Part model, mm, in its own coordinate system. Coordinates: 2 decimals unless noted, no trailing zeros. Loops run counter-clockwise (first coordinate to the right, second up) from the corner with the lowest first, then second, coordinate; pieces in that order, holes last. Notation, with made-up numbers: (19, 84) -> (78, 84) arc R26 ccw to (78, 108) -> close; hole circle Ø1 at (-21.5, 89.25). An arc over 180 degrees is marked (long way). One line per question, with ' | ' between items. Start each with the question number.
1) Cut at B-B (z = 2.25). List the corners of the cut face in (x, y).
2) Probe L1, parallel to Y at x = 27.5, z = 6; L2, parallel to Z at x = 4, y = -88; L3, parallel to Y at x = -20.5, z = 8.25. List the from-to ranges inside material, lowest first. Write a range as from..to.
3) Drop flat-ended pins along their axis: pin 1 (1 mm diameter, centred on x = 6, z = 2, fed in from -Y); pin 2 (4 mm diameter, centred on x = -13, y = -91, fed in from +Z). Give the stop position or say it passes through.
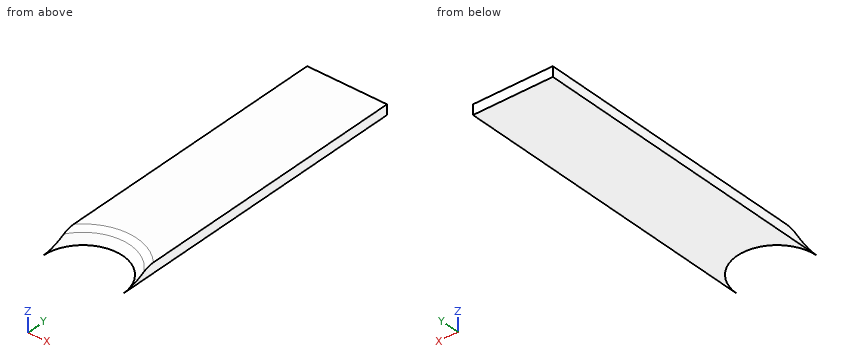
from build123d import *

# Parameters (mm, degrees)
SKETCH1_W           = 80
SKETCH1_H           = 360
BOSS_EXTRUDE1_DEPTH = 10
CUT_EXTRUDE1_DEPTH  = 10
CHAMFER2_SIZE       = 10
FILLET1_R           = 10


with BuildPart() as part:
    # Sketch1 → Boss-Extrude1 (new body)
    with BuildSketch(Plane.XY):
        Rectangle(SKETCH1_W, SKETCH1_H)
    extrude(amount=BOSS_EXTRUDE1_DEPTH)

    # Sketch2 → Cut-Extrude1 (cut)
    with BuildSketch(Plane.XY.offset(10)):
        with BuildLine():
            Line((-40, -135), (-40, -180))
            Line((-40, -180), (40, -180))
            Line((40, -180), (40, -135))
            ThreePointArc((40, -135), (0, -95), (-40, -135))
        make_face()
    extrude(amount=-CUT_EXTRUDE1_DEPTH, mode=Mode.SUBTRACT)

    # Chamfer2
    chamfer2_edges = [part.edges().sort_by_distance(p)[0] for p in [
        (0, -95, 10),
    ]]
    chamfer(chamfer2_edges, length=CHAMFER2_SIZE - 0.0001)  # a hair under: the kernel refuses the full size

    # Fillet1
    fillet1_edges = [part.edges().sort_by_distance(p)[0] for p in [
        (0, -85.0001, 10),
    ]]
    fillet(fillet1_edges, radius=FILLET1_R)


solid = part.part
Reported:
1) outline: (-40, -121.4) arc R42.25 cw to (40, -121.4) -> (40, 180) -> (-40, 180) -> close
2) L1: y = -98.13..180 | L2: z = 0..7.17 | L3: y = -91.06..180
3) pin 1: stops at y = -93.94 | pin 2: stops at z = 7.8
